The listing builds one solid part. Answer for the finished solid, in the listing's coordinates (mm). Coordinates: 2 decimals unless noted, no trailing zeros. Order: outer loops, then holes, each group sorted by start corner. A loop starts at its lowest first (then second) coordinate and runs counter-clockwise, first axis right, second up.
Autodesk Inventor part; units mm, degrees
ref_plane "Work Plane1" through (11.1463, 0, 0) normal (0, 0.7071, -0.7071) x (-1, 0, 0)
ref_plane "YZ Plane" through (0, 0, 0) normal (1, 0, 0) x (0, 1, 0)
ref_plane "XZ Plane" through (0, 0, 0) normal (0, 1, 0) x (-1, 0, 0)
sketch "Skizze1" plane through (0, 0, 0) normal (1, 0, 0) x (0, 1, 0)
  line L0 (0, -3.8891) -> (-3.8891, 0)
  line L1 (-3.8891, 0) -> (0, 3.8891)
  line L2 (0, 3.8891) -> (3.8891, 0)
  line L3 (3.8891, 0) -> (0, -3.8891)
  line L4 (-5.4447, 0) -> (5.4447, 0)
  point P0 (0, 0)
  point P1 (0, 0)
  dimension "d0" = 7.7782
extrude "Körper" add sketch "Skizze1" along normal blind 1.8
sketch "Skizze2" plane through (0, 0, 0) normal (-1, 0, 0) x (0, 0, 1)
  point P0 (0, 0)
  point P1 (0, 0)
hole "Gewinde" at (0, 0, 0) direction (1, 0, 0) diameter 2.459 end through all
chamfer "Fase1" distance 0.2706 angle 30 1 edges at (0, 0, -1.2295) measured on face at (0, -1.5681, 1.6031)
chamfer "Fase2" distance 0.2706 angle 30 1 edges at (1.8, 0, -1.2295) measured on face at (1.8, -1.5681, 1.6031)
ref_plane "Work Plane1" through (11.1463, 0, 0) normal (0, 0.7071, -0.7071) x (-1, 0, 0)
equation "\"d0\" = 1.41421 * SW"
equation "\"d1\" = KOH"
equation "\"d3\" = -0.5 * GD1 + 0.5 * NND"
equation "\"d35\" = -0.5 * GD1 + 0.5 * NND"
equation "\"d5\" = -0.5 * GD1 + 0.5 * NND"
equation "\"d36\" = -0.5 * GD1 + 0.5 * NND"
equation "\"NND\" = 3"
equation "\"KOH\" = 1.8"
equation "\"SW\" = 5.5"
equation "\"GUL\" = 0.541266 * PTC"
equation "\"THREADDIA\" = 3"
equation "\"TOA\" = 30deg"
equation "\"PTC\" = 0.5"
equation "\"E0\" = 7"
equation "\"GAL\" = 0.541266 * PTC"
properties part number "DIN 562 - M3" material "Stahl, weich"
1) A cutting plane is placed at C-C, the plane y = 3.5. Write down the section's boundary in (x, z).
2) The mould has two halves that part along Z. Classify faces 1 (the flat face through (0.89, -1.97, 1.92)), 2 (the cylindrical face through (0.91, 0.748, -0.976)), 3 (the flat face through (0.89, 1.97, -1.92)): released by +Z, released by -Z, zero draft, split by the parting line, or undercut.
3) A cutting plane is placed at B-B, the plane y = -2.25. Write down the section's boundary in (x, z).
4) A cutting plane is placed at A-A, the plane x = 1.25. Write down the section's boundary in (y, z).
5) Straight lines are drawn through the part: probe 1 along Y at (x, z) = (0.8, -0.75); probe 2 along Y at (x, z) = (0.2, -0.5); probe 3 along Y at (x, z) = (0.95, -2). For each, find the intervals that lie inside material, in ascending order.
Working result:
1. outline: (0, -0.39) - (1.8, -0.39) - (1.8, 0.39) - (0, 0.39) - close
2. face 1: released by +Z
2. face 2: undercut
2. face 3: released by -Z
3. outline: (0, -1.64) - (1.8, -1.64) - (1.8, 1.64) - (0, 1.64) - close
4. outline: (-3.89, 0) - (0, -3.89) - (3.89, 0) - (0, 3.89) - close; hole circle Ø2.46 at (0, 0)
5. probe 1: y = -3.14 to -0.97, 0.97 to 3.14
5. probe 2: y = -3.39 to -1.12, 1.12 to 3.39
5. probe 3: y = -1.89 to 1.89
